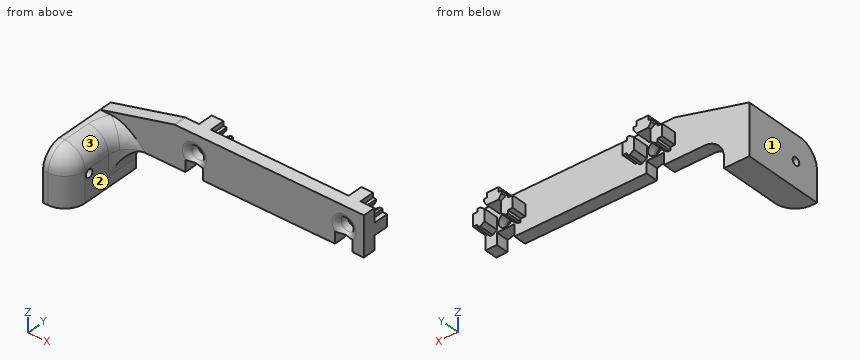
```python
from build123d import *

# Parameters (mm, degrees)
BOSS_EXTRUDE1_DEPTH   = 7.62
BOSS_EXTRUDE1_2_DEPTH = 7.62
BOSS_EXTRUDE1_3_DEPTH = 7.62
BOSS_EXTRUDE1_4_DEPTH = 7.62
SKETCH2_W             = 132.9538108
SKETCH2_H             = 20
BOSS_EXTRUDE2_DEPTH   = 6.35
LPATTERN2_COUNT       = 2
LPATTERN2_PITCH       = 75.4126
CUT_EXTRUDE1_DEPTH    = 125.148300392
FILLET1_R             = 2.54
SKETCH13_R            = 3.5
CUT_EXTRUDE5_DEPTH    = 124.59491895
FILLET6_R             = 2.54
SKETCH14_W            = 8.89
SKETCH14_H            = 5.842
CUT_EXTRUDE6_DEPTH    = 125.148300392
SKETCH15_W            = 25.4
SKETCH15_H            = 40.894
BOSS_EXTRUDE3_DEPTH   = 12.7
FILLET15_R            = 10.16
FILLET16_R            = 10.16
FILLET17_R            = 10.16
FILLET18_R            = 10.16
SKETCH18_R            = 1.984375
CUT_EXTRUDE9_DEPTH    = 12.7


with BuildPart() as part:
    # Sketch1 → Boss-Extrude1 (new body)
    with BuildSketch(Plane(origin=(0, 0, 0), x_dir=(1, 0, 0), z_dir=(0, 1, 0))):
        Polygon((2.9718, 10), (-2.9718, 10), (-2.9718, 7.714), (-4.567901235, 7.714), (-4.567901235, 6.444), (-2.9718, 4.158), (2.9718, 4.158), (4.322098765, 6.444), (4.322098765, 7.714), (2.9718, 7.714), align=None)
    boss_extrude1 = extrude(amount=BOSS_EXTRUDE1_DEPTH)



with BuildPart() as body_2:
    # Sketch1 → Boss-Extrude1 2 (new body)
    with BuildSketch(Plane(origin=(0, 0, 0), x_dir=(1, 0, 0), z_dir=(0, 1, 0))):
        Polygon((4.158, -2.9718), (4.158, 2.9718), (6.444, 4.322098765), (7.714, 4.322098765), (7.714, 2.9718), (10, 2.9718), (10, -2.9718), (7.714, -2.9718), (7.714, -4.567901235), (6.444, -4.567901235), align=None)
    boss_extrude1_2 = extrude(amount=BOSS_EXTRUDE1_2_DEPTH)


with BuildPart() as body_3:
    # Sketch1 → Boss-Extrude1 3 (new body)
    with BuildSketch(Plane(origin=(0, 0, 0), x_dir=(1, 0, 0), z_dir=(0, 1, 0))):
        Polygon((-10, -2.9718), (-10, 2.9718), (-7.714, 2.9718), (-7.714, 4.567901235), (-6.444, 4.567901235), (-4.158, 2.9718), (-4.158, -2.9718), (-6.444, -4.322098765), (-7.714, -4.322098765), (-7.714, -2.9718), align=None)
    boss_extrude1_3 = extrude(amount=BOSS_EXTRUDE1_3_DEPTH)


with BuildPart() as body_4:
    # Sketch1 → Boss-Extrude1 4 (new body)
    with BuildSketch(Plane(origin=(0, 0, 0), x_dir=(1, 0, 0), z_dir=(0, 1, 0))):
        Polygon((4.567901235, -6.444), (2.9718, -4.158), (-2.9718, -4.158), (-4.322098765, -6.444), (-4.322098765, -7.714), (-2.9718, -7.714), (-2.9718, -10), (2.9718, -10), (2.9718, -7.714), (4.567901235, -7.714), align=None)
    boss_extrude1_4 = extrude(amount=BOSS_EXTRUDE1_4_DEPTH)


with BuildPart() as part_1:
    add(part.part)

    add(body_2.part)  # Boss-Extrude2 merges body 2

    add(body_3.part)  # Boss-Extrude2 merges body 3

    add(body_4.part)  # Boss-Extrude2 merges body 4
    # Sketch2 → Boss-Extrude2 (add)
    with BuildSketch(Plane.XZ):
        with Locations((-56.4769054, 0)):
            Rectangle(SKETCH2_W, SKETCH2_H)
    extrude(amount=BOSS_EXTRUDE2_DEPTH)

    # LPattern2: Boss-Extrude1, Boss-Extrude1 2, Boss-Extrude1 3, Boss-Extrude1 4 ×2
    with Locations(*[(-i * LPATTERN2_PITCH, 0, 0) for i in range(1, LPATTERN2_COUNT)]):
        add(boss_extrude1)
        add(boss_extrude1_2)
        add(boss_extrude1_3)
        add(boss_extrude1_4)

    # Sketch4 → Cut-Extrude1 (cut, through all)
    with BuildSketch(Plane(origin=(0, -6.35, 0), x_dir=(-1, 0, 0), z_dir=(0, -1, 0))):
        Polygon((122.9538108, -10), (85.4126108, -10), (122.9538108, -0.2108), align=None)
    extrude(amount=-CUT_EXTRUDE1_DEPTH, mode=Mode.SUBTRACT)

    # Fillet1
    fillet1_edges = [part_1.edges().sort_by_distance(p)[0] for p in [
        (-85.4126108, -3.175, 10),
    ]]
    fillet(fillet1_edges, radius=FILLET1_R)

    # Sketch13 → Cut-Extrude5 (cut, through all)
    with BuildSketch(Plane(origin=(0, 0, 0), x_dir=(1, 0, 0), z_dir=(0, 1, 0))):
        with Locations(Location((0, 0, 0), (0, 0, 270))):
            Circle(SKETCH13_R)
        with Locations(Location((-75.4126, 0, 0), (0, 0, 270))):
            Circle(SKETCH13_R)
    extrude(amount=-CUT_EXTRUDE5_DEPTH, mode=Mode.SUBTRACT)

    # Fillet6
    fillet6_edges = [part_1.edges().sort_by_distance(p)[0] for p in [
        (0, -6.35, -3.5),
        (-75.4126, -6.35, -3.5),
    ]]
    fillet(fillet6_edges, radius=FILLET6_R)

    # Sketch14 → Cut-Extrude6 (cut, through all)
    with BuildSketch(Plane(origin=(0, 7.62, 0), x_dir=(1, 0, 0), z_dir=(0, 1, 0))):
        with Locations((-0.122901235, 7.079)):
            Rectangle(SKETCH14_W, SKETCH14_H)
        with Locations((-75.535501235, 7.079)):
            Rectangle(SKETCH14_W, SKETCH14_H)
    extrude(amount=-CUT_EXTRUDE6_DEPTH, mode=Mode.SUBTRACT)

    # Sketch15 → Boss-Extrude3 (add)
    with BuildSketch(Plane.ZY.offset(122.9538108)):
        with Locations((-12.4892, -20.447)):
            Rectangle(SKETCH15_W, SKETCH15_H)
    extrude(amount=-BOSS_EXTRUDE3_DEPTH)

    # Fillet15
    fillet15_edges = [part_1.edges().sort_by_distance(p)[0] for p in [
        (-110.2538108, -6.35, -4.8946),
    ]]
    fillet(fillet15_edges, radius=FILLET15_R)

    # Fillet16
    fillet16_edges = [part_1.edges().sort_by_distance(p)[0] for p in [
        (-110.2538108, -8.255, -10),
    ]]
    fillet(fillet16_edges, radius=FILLET16_R)

    # Fillet17
    fillet17_edges = [part_1.edges().sort_by_distance(p)[0] for p in [
        (-110.2538108, -40.894, -12.4892),
    ]]
    fillet(fillet17_edges, radius=FILLET17_R)

    # Fillet18
    fillet18_edges = [part_1.edges().sort_by_distance(p)[0] for p in [
        (-107.278015697, -9.325795103, 0.2108),
        (-121.6838108, -40.894, 0.2108),
        (-110.2538108, -23.622, 0.2108),
        (-113.229605903, -37.918204897, 0.2108),
    ]]
    fillet(fillet18_edges, radius=FILLET18_R)

    # Sketch18 → Cut-Extrude9 (cut)
    with BuildSketch(Plane.ZY.offset(122.9538108)):
        with Locations((-12.4892, -28.194)):
            Circle(SKETCH18_R)
    extrude(amount=-CUT_EXTRUDE9_DEPTH, mode=Mode.SUBTRACT)


solid = part_1.part
```
Can you work these out from the model? Positions are in its coordinate system, mm. Face numbers are marked on the shaded views. A direction names the side the tool comes from. Round coordinates to 2 decimals unless told otherwise and drop trailing zeros. Loops run counter-clockwise (first coordinate to the right, second up) from the corner with the lowest first, then second, coordinate; pieces in that order, holes last. Notation, with made-up numbers: M -10.75,73 L 36.25,73 A24 cw 36.25,95 Z; hole C 1,26 d5. An arc over 180 degrees is marked long. Answer as a JSON object with one key per item and string values. Group by question number.
Q1. Please list where these lines run through material, in increasing order: L1, parallel to X at y = -1, z = 0; L2, parallel to X at y = -4, z = -9.5; L3, parallel to Y at x = -57, z = 6.5.
Q2. Imagine slicing it at A-A, the plane x = 0. Please give me the cut outline in (y, z).
Q3. Imagine slicing it at C-C, the plane z = -12. Please give me the cut outline in (x, y).
Q4. Will these pins go through, and if not, where does the flat tip stop? pin 1 (1 mm diameter, centred on y = 4, z = 7, fed in from +X); pin 2 (1.1 mm diameter, centred on x = -4, y = 5, fed in from +Z); pin 3 (2 mm diameter, centred on x = -59, z = -6, fed in from -Y).
Q5. Imagine slicing it at D-D, the plane z = -17.5. Please give me the cut outline in (x, y), then the cut area to 3 significant figures.
Q6. Imagine slicing it at B-B, the plane y = 5. Count the separate pieces of the cut face and the enclosed holes in it, then the cut area to 3 significant figures.
Q7. On a 3-axis mill with a long thin cutter (end or side, diameter ignored), from which of +Z, -Z, +X, -X, +Y, -Y can I reach the whole of each face in a straight line? I mean the marked faces 1, 2 and 3. Say none if no direction works.
Findings:
{
 "1": {"L1": "x = -122.95 to -78.91, -71.91 to -3.5, 3.5 to 10", "L2": "x = -122.95 to -79.98, -71.09 to -4.57, 4.32 to 10", "L3": "y = -6.35 to 0"},
 "2": {"outline": "M -6.35,6.04 A2.54 ccw -3.81,3.5 L 0,3.5 L 0,4.16 L 7.62,4.16 L 7.62,10 L -6.35,10 Z; M -5.52,-4.16 L 0,-4.16 L 0,-3.5 L -3.81,-3.5 A2.54 ccw Z"},
 "3": {"outline": "M -122.95,-40.89 L -120.41,-40.89 A10.16 ccw -110.25,-30.73 L -110.25,-30.12 L -122.95,-30.12 Z; M -122.95,-26.27 L -110.25,-26.27 L -110.25,-16.51 A10.16 cw -106.15,-8.35 L -106.15,0 L -122.95,0 Z"},
 "4": {"pin 1": "stops at x = 4.57", "pin 2": "stops at z = 7.71", "pin 3": "stops at y = -6.35"},
 "5": {"outline": "M -122.95,-40.89 L -120.41,-40.89 A10.16 ccw -110.25,-30.73 L -110.25,-16.51 A10.16 cw -109.9,-13.85 L -109.9,0 L -122.95,0 Z", "area": "502 mm2"},
 "6": {"separate pieces": "6", "enclosed holes": "0", "area": "251 mm2"},
 "7": {"face 1": "+Z, -Z, -X, +Y, -Y", "face 2": "-Z, +X, -Y", "face 3": "+Z, +X, -Y"}
}
